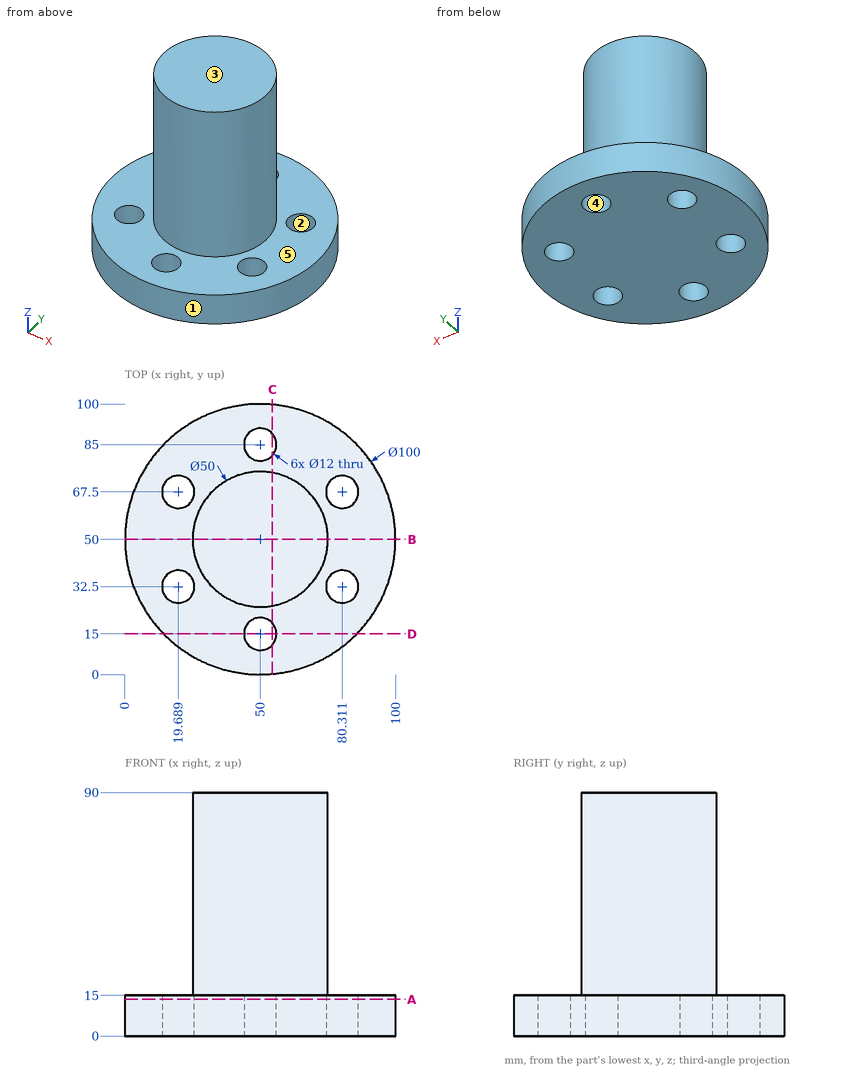
Verification items for this drawing (mm, ordinates from the low corner). A direction names the side the tool comes from. Coordinates: 2 decimals unless noted, no trailing zeros. Loops run counter-clockwise (first coordinate to the right, second up) from the corner with the lowest first, then second, coordinate; pieces in that order, holes last. Notation, with made-up numbers: (-20, 33.25) - (22, 33.25) arc R22 ccw to (22, 42.25) - close; hole circle Ø8 at (49.25, -15.75). An arc over 180 degrees is marked (long way). One line per item, written item: value. Start each with the question number.
(1) Cross-section at D-D on y = 15. Enter the section's corners in (x, z).
(2) Depth check by flat-ended pin: P1, Ø2, axis at y = 56, z = 55.5, coming from the +X side (3 decimals); P2, Ø10, axis at x = 57, z = 76.5, coming from the +Y side; P3, Ø2, axis at x = 68.5, z = 57, coming from the +Y side. Enter the tip coordinate at first touch or a pass-through.
(3) Material ranges on line 1 (Y direction, x = 50, z = 5); line 2 (Z direction, x = 8.5, y = 29.5); line 3 (X direction, y = 67, z = 10), recorded low to high. Write a range as [from, to].
(4) Cross-section at C-C on x = 54.5. Enter the section's corners in (y, z).
(5) Cross-section at B-B on y = 50. Enter the section's corners in (x, z), plus the area to 3 significant figures.
(6) Tool access check on the marked faces 4 and 5. Record the directions out of +Z, -Z, +X, -X, +Y, -Y that give a thin tool (end or side, any length) a straight path to the whole face; none if there is none.
(7) Mould release check, pull along X, two halves, no side actions. Record for the marked faces 1, 2 and 3: released by +X, released by -X, zero draft, split by the parting line, or undercut.
(8) Cross-section at A-A on z = 13.5. Enter the section's corners in (x, y), plus the area to 3 significant figures.
Results below:
1. outline: (14.29, 0) - (44, 0) - (44, 15) - (14.29, 15) - close; (56, 0) - (85.71, 0) - (85.71, 15) - (56, 15) - close
2. P1: stops at x = 74.495
2. P2: stops at y = 74.92
2. P3: stops at y = 67.85
3. line 1: y = [0, 9], [21, 79], [91, 100]
3. line 2: z = [0, 15]
3. line 3: x = [2.98, 13.71], [25.67, 74.33], [86.29, 97.02]
4. outline: (0.2, 0) - (11.03, 0) - (11.03, 15) - (0.2, 15) - close; (18.97, 0) - (81.03, 0) - (81.03, 15) - (74.59, 15) - (74.59, 90) - (25.41, 90) - (25.41, 15) - (18.97, 15) - close; (88.97, 0) - (99.8, 0) - (99.8, 15) - (88.97, 15) - close
5. outline: (0, 0) - (100, 0) - (100, 15) - (75, 15) - (75, 90) - (25, 90) - (25, 15) - (0, 15) - close
5. area: 5,250 mm2
6. face 4: +Z, -Z
6. face 5: +Z
7. face 1: split by the parting line
7. face 2: undercut
7. face 3: zero draft
8. outline: circle Ø100 at (50, 50); hole circle Ø12 at (19.69, 32.5); hole circle Ø12 at (19.69, 67.5); hole circle Ø12 at (50, 15); hole circle Ø12 at (50, 85); hole circle Ø12 at (80.31, 32.5); hole circle Ø12 at (80.31, 67.5)
8. area: 7,180 mm2
